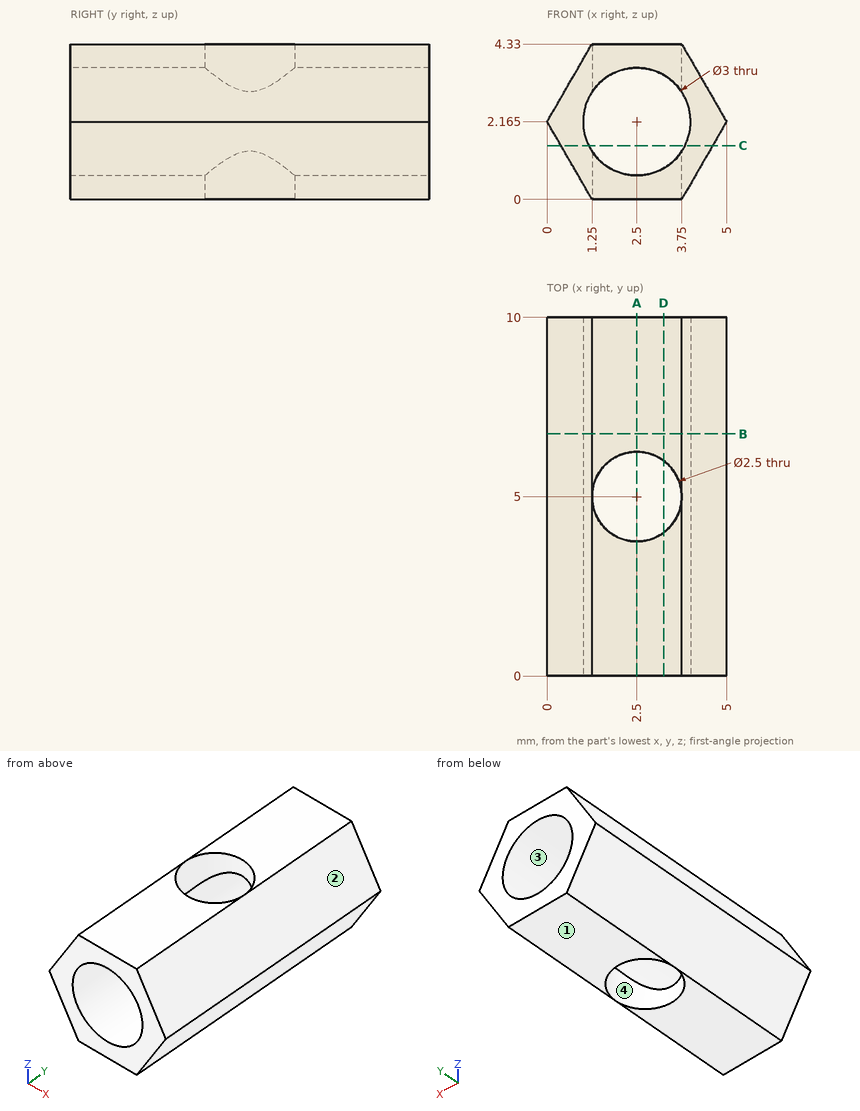
Check sheet for the drawn part. Datum: minimum x, y, z corner. Units: mm. Give positions to 0.01 mm unless a question says otherwise; leave off trailing zeros. Order: outer loops, then holes, each group sorted by start corner. A loop starts at its lowest first (then second) coordinate and runs counter-clockwise, first axis right, second up. Notation, with made-up numbers: (64, 5.5) - (95, 5.5) arc R18 cw to (95, 15.5) - close; hole circle Ø8 at (-40, 20). An arc over 180 degrees is marked (long way). Answer as a JSON object with one key per item and string values.
(1) Cross-section at A-A (x = 2.5). Record the cut outline in (y, z) (3 decimals).
Report:
{"outline": "(0, 0) - (3.75, 0) - (3.75, 0.665) - (0, 0.665) - close; (0, 3.665) - (3.75, 3.665) - (3.75, 4.33) - (0, 4.33) - close; (6.25, 0) - (10, 0) - (10, 0.665) - (6.25, 0.665) - close; (6.25, 3.665) - (10, 3.665) - (10, 4.33) - (6.25, 4.33) - close"}
(2) Cross-section at C-C (z = 1.5). Record the cut outline in (x, y), then the cut area to 3 significant figures.
Report:
{"outline": "(0.38, 0) - (1.16, 0) - (1.16, 10) - (0.38, 10) - close; (3.84, 0) - (4.62, 0) - (4.62, 10) - (3.84, 10) - close", "area": "15.4 mm^2"}
(3) Cross-section at D-D (x = 3.25). Record the cut outline in (y, z).
Report:
{"outline": "(0, 0) - (4, 0) - (4, 0.87) - (0, 0.87) - close; (0, 3.46) - (4, 3.46) - (4, 4.33) - (0, 4.33) - close; (6, 0) - (10, 0) - (10, 0.87) - (6, 0.87) - close; (6, 3.46) - (10, 3.46) - (10, 4.33) - (6, 4.33) - close"}
(4) Draft check along X on the marked faces 1, 2, 3 and 4. Enter one of: released by +X, released by -X, zero draft, split by the parting line, or undercut.
Report:
{"face 1": "zero draft", "face 2": "released by +X", "face 3": "undercut", "face 4": "undercut"}
(5) Material ranges on line 1 (Y direction, x = 2.5, z = 0.4); line 2 (X direction, y = 7.25, z = 1.7); line 3 (Z direction, x = 2.55, y = 0.75), recorded low to high.
Report:
{"line 1": "0 to 3.75, 6.25 to 10", "line 2": "0.27 to 1.07, 3.93 to 4.73", "line 3": "0 to 0.67, 3.66 to 4.33"}
(6) Depth check by flat-ended pin: pin 1 Ø2 at (x, y) = (2.5, 5) entering from +Z; pin 2 Ø1 at (y, z) = (2, 1) entering from +X; pin 3 Ø1.5 at (y, z) = (7, 2) entering from -X; pin 4 Ø1 at (y, z) = (1, 3) entering from +X. Enter the tip coordinate at first touch or a pass-through.
Report:
{"pin 1": "through", "pin 2": "x = 4.62", "pin 3": "x = 0", "pin 4": "x = 4.81"}
(7) Cross-section at B-B (y = 6.75). Record the cut outline in (x, z) (3 decimals).
Report:
{"outline": "(0, 2.165) - (1.25, 0) - (3.75, 0) - (5, 2.165) - (3.75, 4.33) - (1.25, 4.33) - close; hole circle Ø3 at (2.5, 2.165)"}
